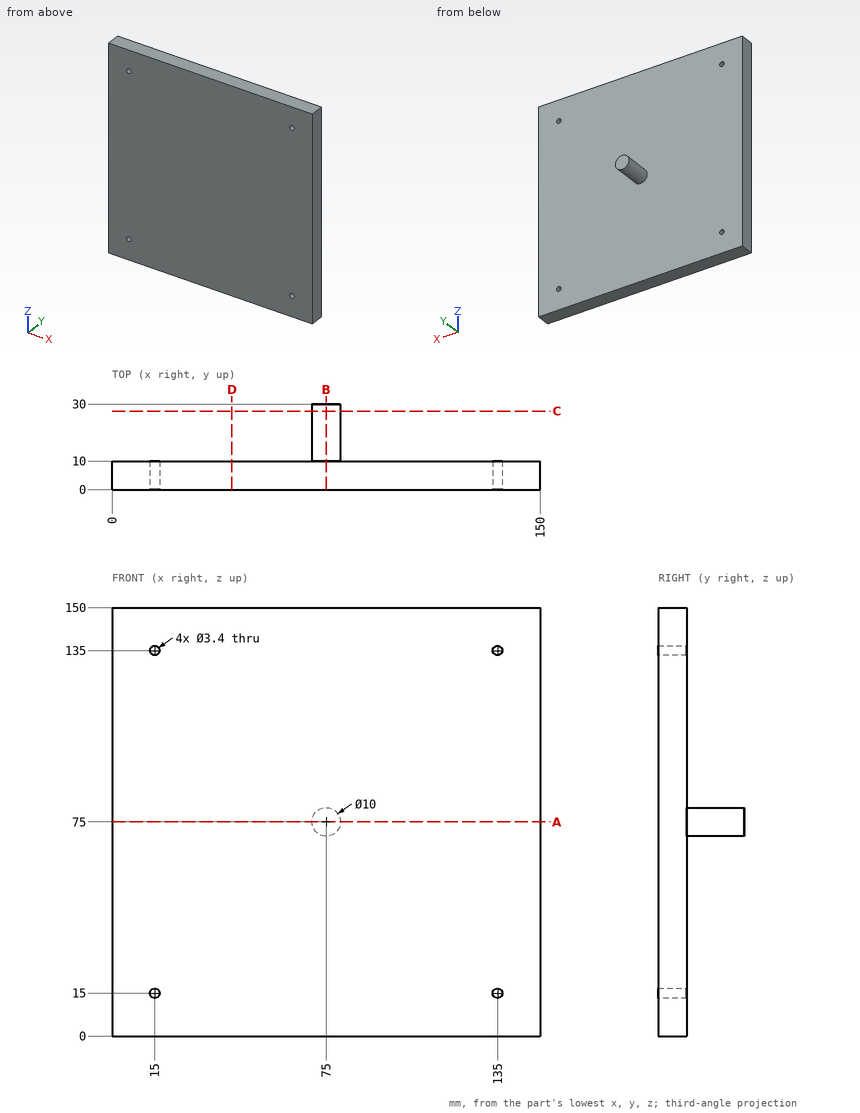
For this review, use the dimensioned drawing (mm, ordinates from the lowest corner) and the shaded views. Coordinates: 2 decimals unless noted, no trailing zeros. Loops run counter-clockwise (first coordinate to the right, second up) from the corner with the lowest first, then second, coordinate; pieces in that order, holes last.
1. For line 1 (Z direction, x = 135, y = 4.75); line 2 (Y direction, x = 40, z = 58), list the stretches that pass through material, from the lowest coordinate up.
2. Add section A-A, the plane z = 75. Give the boundary of the cut face in (x, y), then the cut area to 3 significant figures.
3. Add section B-B, the plane x = 75. Give the boundary of the cut face in (y, z), then the cut area to 3 significant figures.
4. Insertion check: P1, Ø2.5, axis at x = 135, z = 135, coming from the +Y side; P2, Ø10, axis at x = 117.5, z = 56.5, coming from the +Y side; P3, Ø6, axis at x = 79.5, y = 22, coming from the +Z side. Each pin has a flat end and moves straight along its axis. Give the tip position at first contact, or say it passes through.
5. Add section C-C, the plane y = 27.5. Give the boundary of the cut face in (x, z), then the cut area to 3 significant figures.
6. Add section D-D, the plane x = 42. Give the boundary of the cut face in (y, z).
Result:
1. line 1: z = 0 to 13.3, 16.7 to 133.3, 136.7 to 150
1. line 2: y = 0 to 10
2. outline: (0, 0) - (150, 0) - (150, 10) - (80, 10) - (80, 30) - (70, 30) - (70, 10) - (0, 10) - close
2. area: 1,700 mm2
3. outline: (0, 0) - (10, 0) - (10, 70) - (30, 70) - (30, 80) - (10, 80) - (10, 150) - (0, 150) - close
3. area: 1,700 mm2
4. P1: passes through
4. P2: stops at y = 10
4. P3: stops at z = 79.77
5. outline: circle Ø10 at (75, 75)
5. area: 78.5 mm2
6. outline: (0, 0) - (10, 0) - (10, 150) - (0, 150) - close
